```python
from build123d import *

# Parameters (mm, degrees)
BOSS_EXTRUDE1_DEPTH = 100
CUT_EXTRUDE1_DEPTH  = 1001
SKETCH3_R           = 10
CUT_EXTRUDE2_DEPTH  = 1001
FILLET1_R           = 35


with BuildPart() as part:
    # Sketch1 → Boss-Extrude1 (new body, symmetric)
    with BuildSketch(Plane.XY):
        with BuildLine():
            Line((-500, 0), (-500, 80))
            ThreePointArc((-500, 80), (-494.142135624, 94.142135624), (-480, 100))
            Line((-480, 100), (480, 100))
            ThreePointArc((480, 100), (494.142135624, 94.142135624), (500, 80))
            Line((500, 80), (500, 0))
            Line((500, 0), (497, 0))
            Line((497, 0), (497, 80))
            ThreePointArc((497, 80), (492.02081528, 92.02081528), (480, 97))
            Line((480, 97), (-480, 97))
            ThreePointArc((-480, 97), (-492.02081528, 92.02081528), (-497, 80))
            Line((-497, 80), (-497, 0))
            Line((-497, 0), (-500, 0))
        make_face()
    extrude(amount=BOSS_EXTRUDE1_DEPTH, both=True)

    # Sketch2 → Cut-Extrude1 (cut, through all)
    with BuildSketch(Plane(origin=(500, 0, 0), x_dir=(0, 0, -1), z_dir=(1, 0, 0))):
        Polygon((-100, 80), (-100, 0), (-50, 0), align=None)
    extrude(amount=-CUT_EXTRUDE1_DEPTH, mode=Mode.SUBTRACT)

    # Sketch3 → Cut-Extrude2 (cut, through all)
    with BuildSketch(Plane(origin=(500, 0, 0), x_dir=(0, 0, -1), z_dir=(1, 0, 0))):
        with Locations((60, 40)):
            Circle(SKETCH3_R)
    extrude(amount=-CUT_EXTRUDE2_DEPTH, mode=Mode.SUBTRACT)

    # Fillet1
    fillet1_edges = [part.edges().sort_by_distance(p)[0] for p in [
        (498.5, 0, -100),
        (-498.5, 0, -100),
    ]]
    fillet(fillet1_edges, radius=FILLET1_R)


solid = part.part
```
Read the model definition and answer for the solid it produces. Units are mm, in the model's axes. A direction names the side the tool comes from. Coordinates: 2 decimals unless noted, no trailing zeros. Loops run counter-clockwise (first coordinate to the right, second up) from the corner with the lowest first, then second, coordinate; pieces in that order, holes last. Notation, with made-up numbers: (-1, 89) - (55, 89) arc R25 cw to (55, 124) - close; hole circle Ø9 at (-12.5, 31). An arc over 180 degrees is marked (long way). Answer in a Markdown table with one row per item.
1. Given pin 1 (5 mm diameter, centred on y = 89, z = 55.5, fed in from +X); pin 2 (5 mm diameter, centred on y = 83, z = 49, fed in from -X); pin 3 (3 mm diameter, centred on x = -102.5, z = 76.5, fed in from -Y), each flat-ended and moving along its own axis, determine where each tip first touches the part or whether it passes through.
Conclusion:
| item | result |
|---|---|
| pin 1 | stops at x = 498.91 |
| pin 2 | stops at x = -499.99 |
| pin 3 | stops at y = 97 |
2. Determine the mould class of faces 1 (the face through (7, 97, 1)), 2 (the face through (-7, 100, 1)), 3 (the face through (500, 41, 1)), 4 (the face through (-500, 39, 1)) for opening direction X: +X half, -X half, draft (parallel to the pull), parting line (faces both ways), or undercut.
Conclusion:
| item | result |
|---|---|
| face 1 | undercut |
| face 2 | draft |
| face 3 | +X half |
| face 4 | -X half |
3. Straight lines are drawn through the part: line 1 (X direction, y = 31, z = -50); line 2 (Y direction, x = -28, z = 49); line 3 (Y direction, x = 497.85, z = -60). For each, find the intervals that lie inside material, in ascending order.
Conclusion:
| item | result |
|---|---|
| line 1 | x = -500 to -497, 497 to 500 |
| line 2 | y = 97 to 100 |
| line 3 | y = 0 to 30, 50 to 89.02 |
4. Find section A-A, the plane z = 72. Write down the section's boundary in (x, y).
Conclusion:
| item | result |
|---|---|
| outline | (-500, 35.2) - (-497, 35.2) - (-497, 80) arc R17 cw to (-480, 97) - (480, 97) arc R17 cw to (497, 80) - (497, 35.2) - (500, 35.2) - (500, 80) arc R20 ccw to (480, 100) - (-480, 100) arc R20 ccw to (-500, 80) - close |
5. Find section B-B, the plane y = 15. Write down the section's boundary in (x, z) (3 decimals).
Conclusion:
| item | result |
|---|---|
| outline | (-500, -93.723) - (-497, -93.723) - (-497, 59.375) - (-500, 59.375) - close; (497, -93.723) - (500, -93.723) - (500, 59.375) - (497, 59.375) - close |
6. Find section C-C, the plane x = 365. Write down the section's boundary in (y, z).
Conclusion:
| item | result |
|---|---|
| outline | (97, -100) - (100, -100) - (100, 100) - (97, 100) - close |
7. Which of the six approach directions +Z, -Z, +X, -X, +Y, -Y give full straight-line access (tool end or side, diameter ignored) to faces 5 (the face through (-497, 41, 1)), 6 (the face through (499, 34, -52))?
Conclusion:
| item | result |
|---|---|
| face 5 | +Z, -Z, -Y |
| face 6 | +X, -X |
